```python
from build123d import *

# Parameters (mm, degrees)
CROQUIS1_W              = 146
CROQUIS1_H              = 310
SALIENTE_EXTRUIR1_DEPTH = 4
CROQUIS2_W              = 146
CROQUIS2_H              = 2.5
CORTAR_EXTRUIR1_DEPTH   = 10
CROQUIS3_W              = 70
CROQUIS3_H              = 160
CORTAR_EXTRUIR2_DEPTH   = 10


with BuildPart() as part:
    # Croquis1 → Saliente-Extruir1 (new body)
    with BuildSketch(Plane(origin=(0, 0, 0), x_dir=(1, 0, 0), z_dir=(0, 1, 0))):
        with Locations((-123, 0)):
            Rectangle(CROQUIS1_W, CROQUIS1_H)
    extrude(amount=SALIENTE_EXTRUIR1_DEPTH)

    # Croquis2 → Cortar-Extruir1 (cut)
    with BuildSketch(Plane(origin=(0, 4, 0), x_dir=(1, 0, 0), z_dir=(0, 1, 0))):
        with Locations((-123, 153.75)):
            Rectangle(CROQUIS2_W, CROQUIS2_H)
        with Locations((-123, -153.75)):
            Rectangle(CROQUIS2_W, CROQUIS2_H)
    extrude(amount=-CORTAR_EXTRUIR1_DEPTH, mode=Mode.SUBTRACT)

    # Croquis3 → Cortar-Extruir2 (cut)
    with BuildSketch(Plane(origin=(0, 4, 0), x_dir=(1, 0, 0), z_dir=(0, 1, 0))):
        with Locations((-85, 0)):
            Rectangle(CROQUIS3_W, CROQUIS3_H)
    extrude(amount=-CORTAR_EXTRUIR2_DEPTH, mode=Mode.SUBTRACT)


solid = part.part
```
The listing builds one solid part. Answer for the finished solid, in the listing's coordinates (mm). Round coordinates to 2 decimals unless told otherwise and drop trailing zeros. Loops run counter-clockwise (first coordinate to the right, second up) from the corner with the lowest first, then second, coordinate; pieces in that order, holes last. Notation, with made-up numbers: (-25.75, 60) - (23.25, 60) arc R17 ccw to (23.25, 83) - close; hole circle Ø11 at (87.5, -19.75). An arc over 180 degrees is marked (long way). Return JSON: item names as keys, results as strings. Group by question number.
1. The part is cut by section B-B on y = 2.3. Determine the outline of the cut face in (x, z), then the cut area to 3 significant figures.
2. Consider probe 1 along Z at (x, y) = (-106, 0.2); probe 2 along X at (y, z) = (3.6, -39.5). Determine where each line is inside the solid, lowest interval first.
3. This flat-tipped pin is pushed along its axis until it touches: P1, Ø2, axis at y = 1, z = -25, coming from the +X side. Where does it stop, or does it pass through?
4. The part is cut by section C-C on z = -14. Determine the outline of the cut face in (x, y).
5. The part is cut by section A-A on x = -66. Determine the outline of the cut face in (y, z).
Resolved:
{
 "1": {"outline": "(-196, -152.5) - (-50, -152.5) - (-50, -80) - (-120, -80) - (-120, 80) - (-50, 80) - (-50, 152.5) - (-196, 152.5) - close", "area": "33,300 mm²"},
 "2": {"probe 1": "z = -152.5 to -80, 80 to 152.5", "probe 2": "x = -196 to -120"},
 "3": {"P1": "stops at x = -120"},
 "4": {"outline": "(-196, 0) - (-120, 0) - (-120, 4) - (-196, 4) - close"},
 "5": {"outline": "(0, -152.5) - (4, -152.5) - (4, -80) - (0, -80) - close; (0, 80) - (4, 80) - (4, 152.5) - (0, 152.5) - close"}
}
